```python
from build123d import *

# Parameters (mm, degrees)
F1_DEPTH = 2
F3_DEPTH = 5
F5_DEPTH = 3
F6_W     = 3.5266056657
F6_H     = 14.0113048255
F7_DEPTH = 3
F8_SIZE2 = 2.8543093363
F8_SIZE  = 0.3


with BuildPart() as f1:
    # F0 (on Top) → F1 (new body)
    with BuildSketch(Plane.XY):
        with BuildLine():
            Line((37.5, -21), (37.5, 21))
            Line((37.5, 21), (-32.5, 21))
            ThreePointArc((-32.5, 21), (-36.0355339059, 19.5355339059), (-37.5, 16))
            Line((-37.5, 16), (-37.5, -16))
            ThreePointArc((-37.5, -16), (-36.0355339059, -19.5355339059), (-32.5, -21))
            Line((-32.5, -21), (37.5, -21))
        make_face()
    extrude(amount=F1_DEPTH)

    # F2 (on Top) → F3 (join)
    with BuildSketch(Plane.XY):
        with BuildLine():
            ThreePointArc((-36.5, -16), (-35.3284271247, -18.8284271247), (-32.5, -20))
            Line((-32.5, -20), (36.5, -20))
            Line((36.5, -20), (36.5, 20))
            Line((36.5, 20), (-32.5, 20))
            ThreePointArc((-32.5, 20), (-35.3284271247, 18.8284271247), (-36.5, 16))
            Line((-36.5, 16), (-36.5, -16))
        make_face()
    extrude(amount=F3_DEPTH)

    # F4 (on face) → F5 (cut)
    with BuildSketch(Plane.XY.offset(5)):
        with BuildLine():
            ThreePointArc((-32.5, 18), (-33.9142135624, 17.4142135624), (-34.5, 16))
            Line((-34.5, 16), (-34.5, -16))
            ThreePointArc((-34.5, -16), (-33.9142135624, -17.4142135624), (-32.5, -18))
            Line((-32.5, -18), (34.5, -18))
            Line((34.5, -18), (34.5, 18))
            Line((34.5, 18), (-32.5, 18))
        make_face()
    extrude(amount=-F5_DEPTH, mode=Mode.SUBTRACT)

    # F6 (on face) → F7 (cut)
    with BuildSketch(Plane.XY.offset(5)):
        with Locations((-35.1931601763, 0)):
            Rectangle(F6_W, F6_H)
    extrude(amount=-F7_DEPTH, mode=Mode.SUBTRACT)

    # F8
    f8_edges = [f1.edges().sort_by_distance(p)[0] for p in [
        (-36.5, -11.502826, 5),
        (36.5, 0, 5),
        (2, 20, 5),
    ]]
    f8_side = f1.faces().sort_by_distance((2, 19.167594, 5))[0]
    chamfer(f8_edges, length=F8_SIZE, length2=F8_SIZE2, reference=f8_side)


solid = f1.part
```
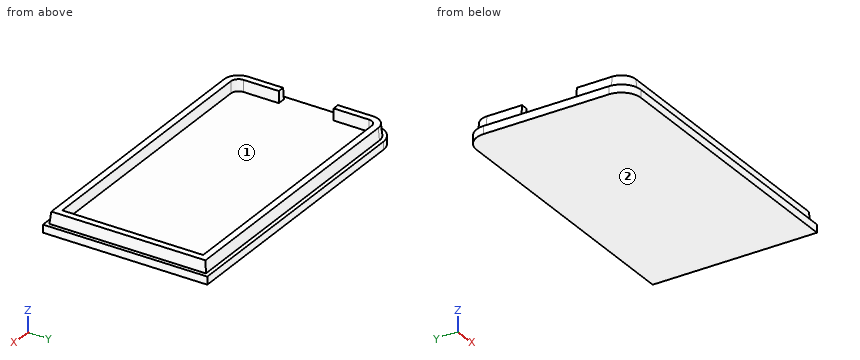
Model file for the job. Use its own axes, mm. Face numbers are marked on the shaded views. Round coordinates to 2 decimals unless told otherwise and drop trailing zeros. Write each loop counter-clockwise with the first axis right and the second up, starting at its lowest first coordinate (ties: lowest second). Pieces come first, ordered by that corner, then holes. Notation, with made-up numbers: (21, -7) -> (48, -7) arc R19 cw to (48, 9) -> close; hole circle Ø9 at (48.25, 35). An arc over 180 degrees is marked (long way). Answer as CSV lines item,"result".
1. Slice it at D-D, the plane y = -2.5. List the corners of the cut face in (x, z), plus the area to 3 significant figures.
Resolved:
outline,"(-37.5, 0) -> (37.5, 0) -> (37.5, 2) -> (36.5, 2) -> (36.5, 2.15) -> (36.2, 5) -> (34.5, 5) -> (34.5, 2) -> (-37.5, 2) -> close"
area,"156 mm²"
2. Mould opens along X. For the marked faces 1 and 2 say: +X half, -X half, draft (parallel to the pull), parting line (faces both ways), or undercut.
Resolved:
face 1,"undercut"
face 2,"draft"
3. Slice it at A-A, the plane y = 10.5. List the corners of the cut face in (x, z), plus the area to 3 significant figures.
Resolved:
outline,"(-37.5, 0) -> (37.5, 0) -> (37.5, 2) -> (36.5, 2) -> (36.5, 2.15) -> (36.2, 5) -> (34.5, 5) -> (34.5, 2) -> (-34.5, 2) -> (-34.5, 5) -> (-36.2, 5) -> (-36.5, 2.15) -> (-36.5, 2) -> (-37.5, 2) -> close"
area,"161 mm²"
4. Pin check, flat tips, straight feed: pin 1 Ø2.5 at (y, z) = (-10, 3) entering from +X; pin 2 Ø1 at (x, z) = (-35, 4) entering from -Y; pin 3 Ø21 at (x, y) = (-10, -3) entering from +Z; pin 4 Ø1.5 at (x, z) = (-3.5, 4) entering from -Y. Stop position of each tip, or through.
Resolved:
pin 1,"x = 37.5"
pin 2,"y = -19.24"
pin 3,"z = 2"
pin 4,"y = -19.88"
5. Slice it at C-C, the plane z = 3.25. List the corners of the cut face in (x, y).
Resolved:
outline,"(-36.38, -16) arc R3.88 ccw to (-32.5, -19.88) -> (36.38, -19.88) -> (36.38, 19.88) -> (-32.5, 19.88) arc R3.88 ccw to (-36.38, 16) -> (-36.38, 7.01) -> (-34.5, 7.01) -> (-34.5, 16) arc R2 cw to (-32.5, 18) -> (34.5, 18) -> (34.5, -18) -> (-32.5, -18) arc R2 cw to (-34.5, -16) -> (-34.5, -7.01) -> (-36.38, -7.01) -> close"
6. Drill centre lines: line 1 (X direction, y = 13, z = 2.25); line 2 (Y direction, x = 0.5, z = 2.1); line 3 (Z direction, x = -16.5, y = -17.5). Where is each one in solid material? Low to high.
Resolved:
line 1,"-36.49 to -34.5, 34.5 to 36.49"
line 2,"-20 to -18, 18 to 20"
line 3,"0 to 2"
7. Slice it at B-B, the plane x = 8. List the corners of the cut face in (y, z), plus the area to 3 significant figures.
Resolved:
outline,"(-21, 0) -> (21, 0) -> (21, 2) -> (20, 2) -> (20, 2.15) -> (19.7, 5) -> (18, 5) -> (18, 2) -> (-18, 2) -> (-18, 5) -> (-19.7, 5) -> (-20, 2.15) -> (-20, 2) -> (-21, 2) -> close"
area,"95.1 mm²"
